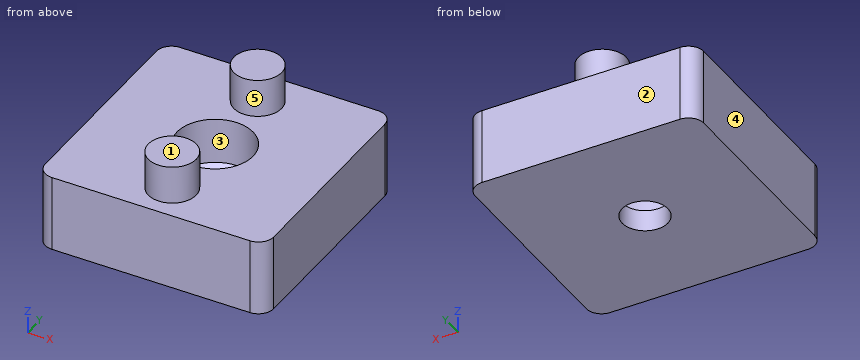
```python
from build123d import *

# Parameters (mm, degrees)
SKETCH005_W    = 30
SKETCH005_H    = 30
PAD003_DEPTH   = 10
SKETCH006_R    = 3.15
PAD004_DEPTH   = 5
SKETCH007_R    = 3
HOLE002_DEPTH  = 25
SKETCH008_R    = 5
HOLE003_DEPTH  = 6
HOLE003_TIPS_R = 5
FILLET_R       = 2


with BuildPart() as part:
    # Sketch005 → Pad003 (new body)
    with BuildSketch(Plane.XY):
        Rectangle(SKETCH005_W, SKETCH005_H)
    extrude(amount=PAD003_DEPTH)

    # Sketch006 (on Face6 of Pad003) → Pad004 (join)
    with BuildSketch(Plane.XY.offset(10)):
        with Locations((0, 10)):
            Circle(SKETCH006_R)
        with Locations((0, -10)):
            Circle(SKETCH006_R)
    extrude(amount=PAD004_DEPTH)

    # Sketch007 (on Face5 of Pad004) → Hole002 (cut)
    with BuildSketch(Plane.XY.offset(10)):
        Circle(SKETCH007_R)
    extrude(amount=-HOLE002_DEPTH, mode=Mode.SUBTRACT)

    # Sketch008 (on Face5 of Hole002) → Hole003 (cut)
    with BuildSketch(Plane.XY.offset(10)):
        Circle(SKETCH008_R)
    extrude(amount=-HOLE003_DEPTH, mode=Mode.SUBTRACT)

    # Hole003 tips → Hole003 tip 1 section 0
    with BuildSketch(Plane.XY.offset(4), mode=Mode.PRIVATE) as hole003_tip_1_s0:
        Circle(HOLE003_TIPS_R)
    loft([hole003_tip_1_s0.sketch, Vertex(0, 0, 0.995697)], mode=Mode.SUBTRACT)

    # Fillet
    fillet_edges = [part.edges().sort_by_distance(p)[0] for p in [
        (15, -15, 5),
        (-15, -15, 5),
        (-15, 15, 5),
        (15, 15, 5),
    ]]
    fillet(fillet_edges, radius=FILLET_R)


with BuildPart() as part_1:
    # Body001 placement: moved
    add(part.part.moved(Location((0, -20, -10))))


solid = part_1.part
```
Input: part model. Units: mm. Frame: model coordinates. Face numbers are marked on the shaded views. A direction names the side the tool comes from. Give positions to 0.01 mm unless a question says otherwise; leave off trailing zeros. Loops run counter-clockwise (first coordinate to the right, second up) from the corner with the lowest first, then second, coordinate; pieces in that order, holes last. Notation, with made-up numbers: M -22,-12 L 19,-12 A20 ccw 19,15 Z; hole C 47.25,-21 d2. An arc over 180 degrees is marked long. Answer as CSV lines item,"result". Start each with the question number.
1. Line query: L1, parallel to Y at x = 0, z = -8.55; L2, parallel to Z at x = 5.25, y = -30.25; L3, parallel to Y at x = 0, z = -2.1. Output: solid intervals per line, ascending.
2. Section C-C on y = -10. Return loops of the section in (x, z), plus the area to 4 significant figures.
3. Reachability of the marked faces 4 and 5 from +Z, -Z, +X, -X, +Y, -Y: full face, straight path, thin tool, end or side. Return the list, or none.
4. Pull-direction query (Y, two-part tool) for the marked faces 1, 2 and 3; classes: released by +Y, released by -Y, zero draft, split by the parting line, or undercut.
5. Section B-B on x = 0. Return loops of the section in (y, z).
6. Pin query (flat end, axial travel): P1, Ø9.5, axis at x = 0, y = -20, coming from the +Z side; P2, Ø5, axis at x = -11.5, y = -19, coming from the +Z side. Return the tip coordinate at first contact, or that it passes through.
7. Section A-A on z = -1. Return loops of the section in (x, y), plus the area to 3 significant figures.
8. Section D-D on x = 6.25. Return loops of the section in (y, z), plus the area to 3 significant figures.
Computed values:
1,L1,"y = -35 to -23, -17 to -5"
1,L2,"z = -10 to 0"
1,L3,"y = -35 to -25, -15 to -5"
2,outline,"M -15,-10 L 15,-10 L 15,0 L 3.15,0 L 3.15,5 L -3.15,5 L -3.15,0 L -15,0 Z"
2,area,"331.5 mm²"
3,face 4,"+Z, -Z, -X, +Y, -Y"
3,face 5,"+Z"
4,face 1,"zero draft"
4,face 2,"released by +Y"
4,face 3,"undercut"
5,outline,"M -35,-10 L -23,-10 L -23,-7.2 L -25,-6 L -25,0 L -26.85,0 L -26.85,5 L -33.15,5 L -33.15,0 L -35,0 Z; M -17,-10 L -5,-10 L -5,0 L -6.85,0 L -6.85,5 L -13.15,5 L -13.15,0 L -15,0 L -15,-6 L -17,-7.2 Z"
6,P1,"stops at z = -6.15"
6,P2,"stops at z = 0"
7,outline,"M -15,-33 A2 ccw -13,-35 L 13,-35 A2 ccw 15,-33 L 15,-7 A2 ccw 13,-5 L -13,-5 A2 ccw -15,-7 Z; hole C 0,-20 d10"
7,area,"818 mm²"
8,outline,"M -35,-10 L -5,-10 L -5,0 L -35,0 Z"
8,area,"300 mm²"
